The listing builds one solid part. Answer for the finished solid, in the listing's coordinates (mm). Round coordinates to 2 decimals unless told otherwise and drop trailing zeros. Write each loop counter-clockwise with the first axis right and the second up, starting at its lowest first coordinate (ties: lowest second). Pieces come first, ordered by that corner, then holes. Notation, with made-up numbers: (62.5, 26) - (88.5, 26) arc R14 ccw to (88.5, 50) - close; hole circle Ø2 at (81, 40). An arc over 180 degrees is marked (long way). Answer in a Markdown table with one row per item.
from build123d import *

# Parameters (mm, degrees)
ESQUISSE2_W             = 201
ESQUISSE2_H             = 75
BOSS_EXTRU_1_DEPTH      = 3
ESQUISSE3_R             = 5
ESQUISSE3_R_2           = 4.999999998
BOSS_EXTRU_3_DEPTH      = 5
BOSS_EXTRU_3_TAPER      = 25
ESQUISSE4_W             = 210
ESQUISSE4_H             = 11.155958732
ENL_V_MAT_EXTRU_1_DEPTH = 2
ESQUISSE5_W             = 220
ESQUISSE5_H             = 18.927618919
ENL_V_MAT_EXTRU_2_DEPTH = 2


with BuildPart() as part:
    # Esquisse2 → Boss.-Extru.1 (new body)
    with BuildSketch(Plane.XY):
        with Locations((0.446886155, -8.200471698)):
            Rectangle(ESQUISSE2_W, ESQUISSE2_H)
    extrude(amount=BOSS_EXTRU_1_DEPTH)

    # Esquisse3 → Boss.-Extru.3 (add)
    with BuildSketch(Plane.XY.offset(3)):
        with Locations((-47.053113845, 9.299528302)):
            Circle(ESQUISSE3_R)
        with Locations((-47.053113845, -40.700471698)):
            Circle(ESQUISSE3_R)
        with Locations((10.946886143, 9.300717009)):
            Circle(ESQUISSE3_R)
        with Locations((10.946886143, -40.699282991)):
            Circle(ESQUISSE3_R)
        with Locations((-86.053113845, 24.299528302)):
            Circle(ESQUISSE3_R)
        with Locations((-56.885494813, 13.799528302)):
            Circle(ESQUISSE3_R)
        with Locations((-86.053113845, 3.299528302)):
            Circle(ESQUISSE3_R)
        with Locations((-86.053113845, -16.700471698)):
            Circle(ESQUISSE3_R)
        with Locations((-86.053113845, -36.700471698)):
            Circle(ESQUISSE3_R)
        with Locations((-61.053113845, -16.700471698)):
            Circle(ESQUISSE3_R_2)
        with Locations((-61.053113845, -36.700471698)):
            Circle(ESQUISSE3_R_2)
        with Locations((86.946886155, 24.299361822)):
            Circle(ESQUISSE3_R)
        with Locations((86.946886155, 3.299528302)):
            Circle(ESQUISSE3_R)
        with Locations((57.779237158, 13.799445062)):
            Circle(ESQUISSE3_R)
        with Locations((86.946886155, -16.700471698)):
            Circle(ESQUISSE3_R)
        with Locations((86.946886155, -36.700471698)):
            Circle(ESQUISSE3_R)
        with Locations((61.946886155, -36.700471698)):
            Circle(ESQUISSE3_R)
        with Locations((61.946886155, -16.700471698)):
            Circle(ESQUISSE3_R)
    extrude(amount=BOSS_EXTRU_3_DEPTH, taper=BOSS_EXTRU_3_TAPER)

    # Esquisse4 → Enlèv. mat.-Extru.1 (cut)
    with BuildSketch(Plane(origin=(0, 29.299528302, 0), x_dir=(1, 0, 0), z_dir=(0, 1, 0))):
        with Locations((1.418471148, -5.577979366)):
            Rectangle(ESQUISSE4_W, ESQUISSE4_H)
    extrude(amount=-ENL_V_MAT_EXTRU_1_DEPTH, mode=Mode.SUBTRACT)

    # Esquisse5 → Enlèv. mat.-Extru.2 (cut)
    with BuildSketch(Plane(origin=(0, -45.700471698, 0), x_dir=(-1, 0, 0), z_dir=(0, -1, 0))):
        with Locations((0.053113845, -9.46380946)):
            Rectangle(ESQUISSE5_W, ESQUISSE5_H)
    extrude(amount=-ENL_V_MAT_EXTRU_2_DEPTH, mode=Mode.SUBTRACT)


solid = part.part
(1) Find the intervals of material crossed by line 1 (X direction, y = -16, z = 7.25); line 2 (X direction, y = -15.5, z = 5.25); line 3 (X direction, y = -39, z = 5.5), in increasing order.
Checked values:
| item | result |
|---|---|
| line 1 | x = -88.99 to -83.12, -63.99 to -58.12, 59.01 to 64.88, 84.01 to 89.88 |
| line 2 | x = -89.82 to -82.29, -64.82 to -57.29, 58.18 to 65.71, 83.18 to 90.71 |
| line 3 | x = -89.12 to -82.98, -64.12 to -57.98, -50.49 to -43.62, 7.51 to 14.38, 58.88 to 65.02, 83.88 to 90.02 |
(2) A flat-ended cylindrical pin translates along its axis: pin 1 (3 mm diameter, centred on x = 77, y = 16, fed in from +Z). Find the tip coordinate at first contact, or state that the pin passes through.
Checked values:
| item | result |
|---|---|
| pin 1 | stops at z = 3 |
(3) Section C-C (x = 23.5) is taken. Give the vertices of the cut face in (y, z), and give its area (3 significant figures).
Checked values:
| item | result |
|---|---|
| outline | (-43.7, 0) - (27.3, 0) - (27.3, 3) - (-43.7, 3) - close |
| area | 213 mm2 |
(4) Section B-B (y = -23.5) is taken. Give the vertices of the cut face in (x, z), and give its area (3 significant figures).
Checked values:
| item | result |
|---|---|
| outline | (-100.05, 0) - (100.95, 0) - (100.95, 3) - (-100.05, 3) - close |
| area | 603 mm2 |
(5) Section A-A (z = 4.25) is taken. State how many separate pieces and enclosed holes the cut face has, and give its area (3 significant figures).
Checked values:
| item | result |
|---|---|
| separate pieces | 18 |
| enclosed holes | 0 |
| area | 1,080 mm2 |
